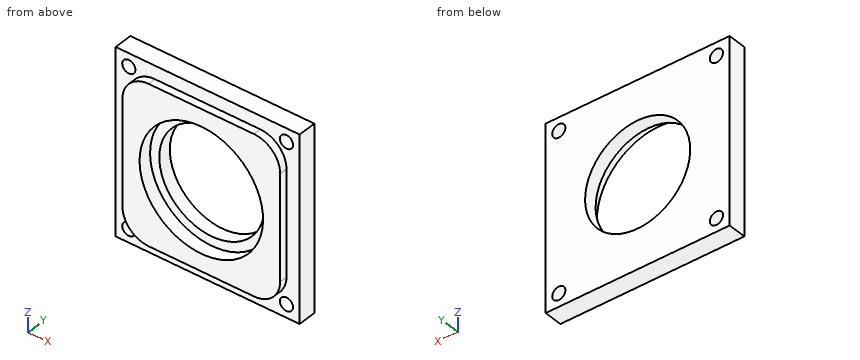
from build123d import *

# Parameters (mm, degrees)
SZKIC1_W                    = 70
SZKIC1_H                    = 70
SZKIC1_R                    = 20
SZKIC1_R_2                  = 2.5
DODANIE_WYCI_GNI_CIE1_DEPTH = 10
SZKIC1_3_W                  = 70
SZKIC1_3_H                  = 70
WYTNIJ_WYCI_GNI_CIE1_DEPTH  = 3
SZKIC1_4_R                  = 23.5
SZKIC1_4_R_2                = 20
WYTNIJ_WYCI_GNI_CIE2_DEPTH  = 5


with BuildPart() as part:
    # Szkic1 → Dodanie-wyci_gni_cie1 (new body)
    with BuildSketch(Plane(origin=(0, 0, 0), x_dir=(1, 0, 0), z_dir=(0, 1, 0))):
        with Locations((35, 35)):
            Rectangle(SZKIC1_W, SZKIC1_H)
        with Locations(Location((35, 35, 0), (0, 0, 270))):
            Circle(SZKIC1_R, mode=Mode.SUBTRACT)
        with Locations(Location((5, 5, 0), (0, 0, 270))):
            Circle(SZKIC1_R_2, mode=Mode.SUBTRACT)
        with Locations(Location((65, 5, 0), (0, 0, 270))):
            Circle(SZKIC1_R_2, mode=Mode.SUBTRACT)
        with Locations(Location((65, 65, 0), (0, 0, 270))):
            Circle(SZKIC1_R_2, mode=Mode.SUBTRACT)
        with Locations(Location((5, 65, 0), (0, 0, 270))):
            Circle(SZKIC1_R_2, mode=Mode.SUBTRACT)
    extrude(amount=DODANIE_WYCI_GNI_CIE1_DEPTH)

    # Szkic1_3 → Wytnij-wyci_gni_cie1 (cut)
    with BuildSketch(Plane(origin=(0, 0, 0), x_dir=(1, 0, 0), z_dir=(0, 1, 0))):
        with Locations((35, 35)):
            Rectangle(SZKIC1_3_W, SZKIC1_3_H)
        with BuildLine():
            Line((5, 35), (5, 55))
            ThreePointArc((5, 55), (7.928932188, 62.071067812), (15, 65))
            Line((15, 65), (55, 65))
            ThreePointArc((55, 65), (62.071067812, 62.071067812), (65, 55))
            Line((65, 55), (65, 15))
            ThreePointArc((65, 15), (62.071067812, 7.928932188), (55, 5))
            Line((55, 5), (15, 5))
            ThreePointArc((15, 5), (7.928932188, 7.928932188), (5, 15))
            Line((5, 15), (5, 35))
        make_face(mode=Mode.SUBTRACT)
    extrude(amount=WYTNIJ_WYCI_GNI_CIE1_DEPTH, mode=Mode.SUBTRACT)

    # Szkic1_4 → Wytnij-wyci_gni_cie2 (cut)
    with BuildSketch(Plane(origin=(0, 0, 0), x_dir=(1, 0, 0), z_dir=(0, 1, 0))):
        with Locations(Location((35, 35, 0), (0, 0, 270))):
            Circle(SZKIC1_4_R)
        with Locations(Location((35, 35, 0), (0, 0, 270))):
            Circle(SZKIC1_4_R_2, mode=Mode.SUBTRACT)
    extrude(amount=WYTNIJ_WYCI_GNI_CIE2_DEPTH, mode=Mode.SUBTRACT)


solid = part.part
Geometry check sheet. Reference: the model listing, model coordinates, mm. Coordinates: 2 decimals unless noted, no trailing zeros. Loops run counter-clockwise (first coordinate to the right, second up) from the corner with the lowest first, then second, coordinate; pieces in that order, holes last. Notation, with made-up numbers: (52.25, 28) - (88.25, 28) arc R27 ccw to (88.25, 60) - close; hole circle Ø4 at (-29.5, 35). An arc over 180 degrees is marked (long way). Use one line per item in the form item = value. Start each with the question number.
Item 1: Gauge pin test, flat ends, axial feed: pin 1 (3.5 mm diameter, centred on x = 31, y = 1, fed in from -Z); pin 2 (4 mm diameter, centred on x = 65, z = -5, fed in from +Y); pin 3 (1.5 mm diameter, centred on y = 1, z = -25.5, fed in from +X); pin 4 (1.5 mm diameter, centred on x = 28.5, y = 1, fed in from +Z). Record the tip position at first contact, or that the pin passes through.
Item 2: Section check C-C, the plane x = 35. Enter the section's corners in (y, z).
Item 3: Section check A-A, the plane z = -35. Enter the section's corners in (x, y).
Item 4: Section check B-B, the plane y = 9. Enter the section's corners in (x, z), and give its area (3 significant figures).
Item 5: Thickness scan on probe 1 along X at (y, z) = (5.25, -5); probe 2 along Z at (x, y) = (65, 8.25); probe 3 along X at (y, z) = (1.5, -35). Record the ranges inside material, lowest first.
Item 6: Section check D-D, the plane y = 1.75. Enter the section's corners in (x, z).
Computed:
q1.pin_1 = -65
q1.pin_2 = through
q1.pin_3 = 65
q1.pin_4 = -5
q2.outline = (0, -65) - (3, -65) - (3, -70) - (10, -70) - (10, -55) - (5, -55) - (5, -58.5) - (0, -58.5) - close; (0, -11.5) - (5, -11.5) - (5, -15) - (10, -15) - (10, 0) - (3, 0) - (3, -5) - (0, -5) - close
q3.outline = (0, 3) - (5, 3) - (5, 0) - (11.5, 0) - (11.5, 5) - (15, 5) - (15, 10) - (0, 10) - close; (55, 5) - (58.5, 5) - (58.5, 0) - (65, 0) - (65, 3) - (70, 3) - (70, 10) - (55, 10) - close
q4.outline = (0, -70) - (70, -70) - (70, 0) - (0, 0) - close; hole circle Ø5 at (5, -65); hole circle Ø5 at (5, -5); hole circle Ø40 at (35, -35); hole circle Ø5 at (65, -65); hole circle Ø5 at (65, -5)
q4.area = 3,560 mm2
q5.probe_1 = 0 to 2.5, 7.5 to 62.5, 67.5 to 70
q5.probe_2 = -70 to -67.5, -62.5 to -7.5, -2.5 to 0
q5.probe_3 = 5 to 11.5, 58.5 to 65
q6.outline = (5, -55) arc R10 ccw to (15, -65) - (55, -65) arc R10 ccw to (65, -55) - (65, -15) arc R10 ccw to (55, -5) - (15, -5) arc R10 ccw to (5, -15) - close; hole circle Ø47 at (35, -35)
